```python
from build123d import *

# Parameters (mm, degrees)
F2_R     = 3.8646706833
F3_DEPTH = 203.2
F4_R     = 5.08
F5_W     = 3.5796575248
F5_H     = 2.878639847
F6_DEPTH = 25.4


with BuildPart() as f1:
    # F0 (on Right) → F1 (revolve)
    with BuildSketch(Plane.YZ):
        with BuildLine():
            add(Edge.make_bspline(
                [(-76.579041779, 18.8016630709), (-69.1488949828, 15.6394448175), (-52.4087731855, 8.5149666392), (-13.3308835609, 22.6696192437), (25.1879196064, 8.4129311715), (62.5127613012, 17.479987921), (72.2691334601, 11.5001326867), (76.0300904512, 9.1949747875)],
                knots=[0, 0, 0, 0, 0.1813555958, 0.4085941832, 0.64367127, 0.8626398208, 1, 1, 1, 1], degree=3))
            Line((-76.579041779, 18.8016630709), (-75.4811316729, 0))
            Line((-75.4811316729, 0), (75.2066522837, 0))
            Line((75.2066522837, 0), (76.0300904512, 9.1949747875))
        make_face()
    revolve(axis=Axis((0, -0.1372396946, 0), (0, 1, 0)))

    # F2 (on Front) → F3 (join)
    with BuildSketch(Plane.XZ):
        Circle(F2_R)
    extrude(amount=F3_DEPTH)

    # F4
    f4_edges = [f1.edges().sort_by_distance(p)[0] for p in [
        (0, -76.579042, -18.801663),
    ]]
    fillet(f4_edges, radius=F4_R)

    # F5 (on face) → F6 (join)
    with BuildSketch(Plane.XZ.offset(203.2)):
        Rectangle(F5_W, F5_H)
    extrude(amount=F6_DEPTH)


solid = f1.part
```
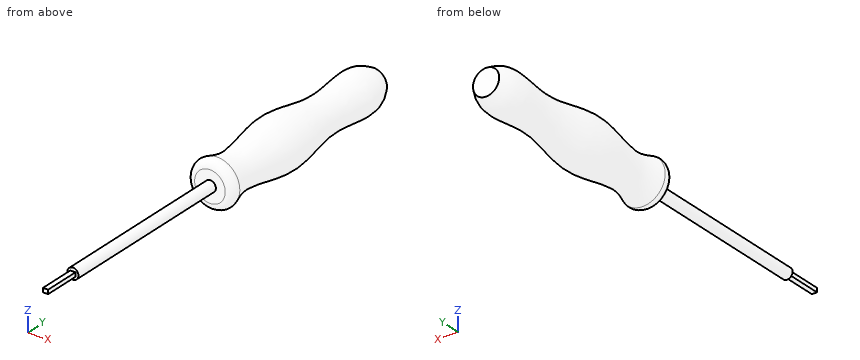
CAD build for the part. Positions are in the model's coordinates, mm. Give positions to 0.01 mm unless a question says otherwise; leave off trailing zeros. Loops run counter-clockwise (first coordinate to the right, second up) from the corner with the lowest first, then second, coordinate; pieces in that order, holes last. Notation, with made-up numbers: (-11, -24) - (36, -24) arc R29 ccw to (36, 15) - close; hole circle Ø8 at (-35, 66.5). An arc over 180 degrees is marked (long way). Put each result on its own line as item: value.
Q1. Flat gauge pins, fed straight in: pin 1 (0.9 mm diameter, centred on y = -217, z = 0, fed in from -X); pin 2 (12 mm diameter, centred on y = -198, z = 3, fed in from +X); pin 3 (10 mm diameter, centred on x = 13.5, z = 13.5, fed in from -Y). Where does each tip first touch, or does it go through?
Filled in:
pin 1: stops at x = -1.79
pin 2: stops at x = 3.86
pin 3: stops at y = -75.12
Q2. Probe line 1 along X through (y, z) = (-133, 0); line 2 along X through (y, z) = (-99, -1); line 3 along Y through (x, z) = (-2, 4). List the from-to ranges inside material, lowest first.
Filled in:
line 1: x = -3.86 to 3.86
line 2: x = -3.73 to 3.73
line 3: y = -75.74 to 75.61
Q3. Slice it at A-A (y = -148.5). Give the cut face in (x, z), plus the area to 3 significant figures.
Filled in:
outline: circle Ø7.73 at (0, 0)
area: 46.9 mm²
